Work out the finished part from the listing and answer in its coordinate system (mm). Give positions to 0.01 mm unless a question says otherwise; leave off trailing zeros.
1) Given pin 1 Ø1.1 at (x, z) = (0.5, 48.5) entering from +Y; pin 2 Ø1 at (y, z) = (7.5, -7.5) entering from +X, each flat-ended and moving along its own axis, determine where each tip first touches the part or whether it passes through.
2) Find section A-A (z = -72). Count the separate pieces of the cut face and the enclosed holes in it, plus the area to 3 significant figures.
3) Straight lines are drawn through the part: probe 1 along X at (y, z) = (-3.25, -44); probe 2 along X at (y, z) = (-5.5, -96); probe 3 along Y at (x, z) = (13.5, 64.5) (3 decimals). For each, find the intervals that lie inside material, in ascending order.
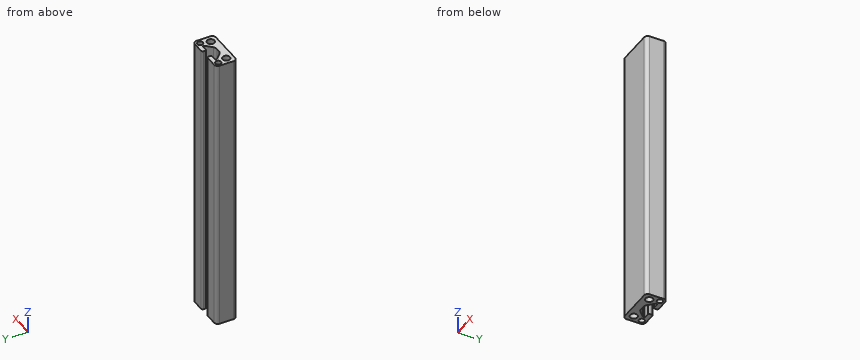
```python
from build123d import *

# Parameters (mm, degrees)
SKETCH2_R           = 2.5527
SKETCH2_R_2         = 3.3274
BOSS_EXTRUDE1_DEPTH = 126.785


with BuildPart() as part:
    # Sketch2 → Boss-Extrude1 (new, symmetric)
    with BuildSketch(Plane.XY):
        with BuildLine():
            Line((-10.287, 4.255364987), (-10.287, 4.572))
            ThreePointArc((-10.287, 4.572), (-10.026617928, 5.200617928), (-9.398, 5.461))
            Line((-9.398, 5.461), (-5.334, 5.461))
            ThreePointArc((-5.334, 5.461), (-4.435974388, 5.832974388), (-4.064, 6.731))
            Line((-4.064, 6.731), (-4.064, 8.001))
            ThreePointArc((-4.064, 8.001), (-4.510369265, 9.078630735), (-5.588, 9.525))
            Line((-5.588, 9.525), (-15.875, 9.525))
            ThreePointArc((-15.875, 9.525), (-18.12006403, 8.59506403), (-19.05, 6.35))
            Line((-19.05, 6.35), (-19.05, -6.35))
            ThreePointArc((-19.05, -6.35), (-18.12006403, -8.59506403), (-15.875, -9.525))
            Line((-15.875, -9.525), (15.875, -9.525))
            ThreePointArc((15.875, -9.525), (18.12006403, -8.59506403), (19.05, -6.35))
            Line((19.05, -6.35), (19.05, 6.35))
            ThreePointArc((19.05, 6.35), (18.12006403, 8.59506403), (15.875, 9.525))
            Line((15.875, 9.525), (5.588, 9.525))
            ThreePointArc((5.588, 9.525), (4.510369265, 9.078630735), (4.064, 8.001))
            Line((4.064, 8.001), (4.064, 6.731))
            ThreePointArc((4.064, 6.731), (4.435974388, 5.832974388), (5.334, 5.461))
            Line((5.334, 5.461), (9.398, 5.461))
            ThreePointArc((9.398, 5.461), (10.026617928, 5.200617928), (10.287, 4.572))
            Line((10.287, 4.572), (10.287, 4.255364987))
            ThreePointArc((10.287, 4.255364987), (10.219328904, 3.915159416), (10.026617928, 3.626747059))
            Line((10.026617928, 3.626747059), (5.124055081, -1.275815789))
            ThreePointArc((5.124055081, -1.275815789), (3.583109058, -2.305443004), (1.765439291, -2.667))
            Line((1.765439291, -2.667), (-1.765439291, -2.667))
            ThreePointArc((-1.765439291, -2.667), (-3.583109058, -2.305443004), (-5.124055081, -1.275815789))
            Line((-5.124055081, -1.275815789), (-10.026617928, 3.626747059))
            ThreePointArc((-10.026617928, 3.626747059), (-10.219328904, 3.915159416), (-10.287, 4.255364987))
        make_face()
        with Locations((-14.848796959, 5.276432773)):
            Circle(SKETCH2_R, mode=Mode.SUBTRACT)
        with Locations((-12.7, -3.175)):
            Circle(SKETCH2_R_2, mode=Mode.SUBTRACT)
        with Locations((12.7, -3.175)):
            Circle(SKETCH2_R_2, mode=Mode.SUBTRACT)
        with Locations((14.848796959, 5.276432773)):
            Circle(SKETCH2_R, mode=Mode.SUBTRACT)
    extrude(amount=BOSS_EXTRUDE1_DEPTH, both=True)


solid = part.part
```
Results:
1. pin 1: stops at y = -2.67
1. pin 2: stops at x = 18.98
2. separate pieces: 1
2. enclosed holes: 4
2. area: 449 mm2
3. probe 1: x = -19.05 to -16.03, -9.37 to 9.37, 16.03 to 19.05
3. probe 2: x = -19.05 to -15.08, -10.32 to 10.32, 15.08 to 19.05
3. probe 3: y = -9.525 to -6.405, 0.055 to 3.109, 7.444 to 9.525
